```python
from build123d import *

# Parameters (mm, degrees)
SKETCH2_R           = 2.1
BOSS_EXTRUDE1_DEPTH = 746


with BuildPart() as part:
    # Sketch2 → Boss-Extrude1 (new body)
    with BuildSketch(Plane.XY):
        with BuildLine():
            Line((-0.1, 3.9), (0, 3.8))
            Line((0, 3.8), (0.1, 3.9))
            Line((0.1, 3.9), (2.840365134, 3.9))
            Line((2.840365134, 3.9), (5.5, 6.558825842))
            Line((5.5, 6.558825842), (5.5, 8.197505675))
            Line((5.5, 8.197505675), (2.89, 8.197505675))
            Line((2.89, 8.197505675), (2.89, 8.307505675))
            Line((2.89, 8.307505675), (4.348614357, 9.766120032))
            ThreePointArc((4.348614357, 9.766120032), (4.604908803, 9.937370505), (4.907228714, 9.997505675))
            Line((4.907228714, 9.997505675), (8.5, 9.997505675))
            ThreePointArc((8.5, 9.997505675), (9.560660172, 9.558165846), (10, 8.497505675))
            Line((10, 8.497505675), (10, 4.904734389))
            ThreePointArc((10, 4.904734389), (9.939864831, 4.602414477), (9.768614357, 4.346120032))
            Line((9.768614357, 4.346120032), (8.31, 2.887505675))
            Line((8.31, 2.887505675), (8.2, 2.887505675))
            Line((8.2, 2.887505675), (8.2, 5.497505675))
            Line((8.2, 5.497505675), (6.56, 5.497505675))
            Line((6.56, 5.497505675), (3.9, 2.83831481))
            Line((3.9, 2.83831481), (3.9, 0.1))
            Line((3.9, 0.1), (3.8, 0))
            Line((3.8, 0), (3.9, -0.1))
            Line((3.9, -0.1), (3.9, -2.84))
            Line((3.9, -2.84), (6.56, -5.5))
            Line((6.56, -5.5), (8.2, -5.5))
            Line((8.2, -5.5), (8.2, -2.89))
            Line((8.2, -2.89), (8.31, -2.89))
            Line((8.31, -2.89), (9.765685425, -4.345685425))
            ThreePointArc((9.765685425, -4.345685425), (9.939103626, -4.605224104), (10, -4.91137085))
            Line((10, -4.91137085), (10, -15.08862915))
            ThreePointArc((10, -15.08862915), (9.939103626, -15.394775896), (9.765685425, -15.654314575))
            Line((9.765685425, -15.654314575), (8.31, -17.11))
            Line((8.31, -17.11), (8.2, -17.11))
            Line((8.2, -17.11), (8.2, -14.5))
            Line((8.2, -14.5), (6.56, -14.5))
            Line((6.56, -14.5), (3.9, -17.16))
            Line((3.9, -17.16), (3.9, -19.9))
            Line((3.9, -19.9), (3.8, -20))
            Line((3.8, -20), (3.9, -20.1))
            Line((3.9, -20.1), (3.9, -22.83831481))
            Line((3.9, -22.83831481), (6.56, -25.497505675))
            Line((6.56, -25.497505675), (8.2, -25.497505675))
            Line((8.2, -25.497505675), (8.2, -22.887505675))
            Line((8.2, -22.887505675), (8.31, -22.887505675))
            Line((8.31, -22.887505675), (9.768614357, -24.346120032))
            ThreePointArc((9.768614357, -24.346120032), (9.939864831, -24.602414477), (10, -24.904734389))
            Line((10, -24.904734389), (10, -28.497505675))
            ThreePointArc((10, -28.497505675), (9.560660172, -29.558165846), (8.5, -29.997505675))
            Line((8.5, -29.997505675), (4.907228714, -29.997505675))
            ThreePointArc((4.907228714, -29.997505675), (4.604908803, -29.937370505), (4.348614357, -29.766120032))
            Line((4.348614357, -29.766120032), (2.89, -28.307505675))
            Line((2.89, -28.307505675), (2.89, -28.197505675))
            Line((2.89, -28.197505675), (5.5, -28.197505675))
            Line((5.5, -28.197505675), (5.5, -26.558825842))
            Line((5.5, -26.558825842), (2.840365134, -23.9))
            Line((2.840365134, -23.9), (0.1, -23.9))
            Line((0.1, -23.9), (0, -23.8))
            Line((0, -23.8), (-0.1, -23.9))
            Line((-0.1, -23.9), (-2.840365134, -23.9))
            Line((-2.840365134, -23.9), (-5.5, -26.558825842))
            Line((-5.5, -26.558825842), (-5.5, -28.197505675))
            Line((-5.5, -28.197505675), (-2.89, -28.197505675))
            Line((-2.89, -28.197505675), (-2.89, -28.307505675))
            Line((-2.89, -28.307505675), (-4.348614357, -29.766120032))
            ThreePointArc((-4.348614357, -29.766120032), (-4.604908803, -29.937370505), (-4.907228714, -29.997505675))
            Line((-4.907228714, -29.997505675), (-8.5, -29.997505675))
            ThreePointArc((-8.5, -29.997505675), (-9.560660172, -29.558165846), (-10, -28.497505675))
            Line((-10, -28.497505675), (-10, -24.904734389))
            ThreePointArc((-10, -24.904734389), (-9.939864831, -24.602414477), (-9.768614357, -24.346120032))
            Line((-9.768614357, -24.346120032), (-8.31, -22.887505675))
            Line((-8.31, -22.887505675), (-8.2, -22.887505675))
            Line((-8.2, -22.887505675), (-8.2, -25.497505675))
            Line((-8.2, -25.497505675), (-6.56, -25.497505675))
            Line((-6.56, -25.497505675), (-3.9, -22.83831481))
            Line((-3.9, -22.83831481), (-3.9, -20.1))
            Line((-3.9, -20.1), (-3.8, -20))
            Line((-3.8, -20), (-3.9, -19.9))
            Line((-3.9, -19.9), (-3.9, -17.16))
            Line((-3.9, -17.16), (-6.56, -14.5))
            Line((-6.56, -14.5), (-8.2, -14.5))
            Line((-8.2, -14.5), (-8.2, -17.11))
            Line((-8.2, -17.11), (-8.31, -17.11))
            Line((-8.31, -17.11), (-9.765685425, -15.654314575))
            ThreePointArc((-9.765685425, -15.654314575), (-9.939103626, -15.394775896), (-10, -15.08862915))
            Line((-10, -15.08862915), (-10, -4.91137085))
            ThreePointArc((-10, -4.91137085), (-9.939103626, -4.605224104), (-9.765685425, -4.345685425))
            Line((-9.765685425, -4.345685425), (-8.31, -2.89))
            Line((-8.31, -2.89), (-8.2, -2.89))
            Line((-8.2, -2.89), (-8.2, -5.5))
            Line((-8.2, -5.5), (-6.56, -5.5))
            Line((-6.56, -5.5), (-3.9, -2.84))
            Line((-3.9, -2.84), (-3.9, -0.1))
            Line((-3.9, -0.1), (-3.8, 0))
            Line((-3.8, 0), (-3.9, 0.1))
            Line((-3.9, 0.1), (-3.9, 2.83831481))
            Line((-3.9, 2.83831481), (-6.56, 5.497505675))
            Line((-6.56, 5.497505675), (-8.2, 5.497505675))
            Line((-8.2, 5.497505675), (-8.2, 2.887505675))
            Line((-8.2, 2.887505675), (-8.31, 2.887505675))
            Line((-8.31, 2.887505675), (-9.768614357, 4.346120032))
            ThreePointArc((-9.768614357, 4.346120032), (-9.939864831, 4.602414477), (-10, 4.904734389))
            Line((-10, 4.904734389), (-10, 8.497505675))
            ThreePointArc((-10, 8.497505675), (-9.560660172, 9.558165846), (-8.5, 9.997505675))
            Line((-8.5, 9.997505675), (-4.907228714, 9.997505675))
            ThreePointArc((-4.907228714, 9.997505675), (-4.604908803, 9.937370505), (-4.348614357, 9.766120032))
            Line((-4.348614357, 9.766120032), (-2.89, 8.307505675))
            Line((-2.89, 8.307505675), (-2.89, 8.197505675))
            Line((-2.89, 8.197505675), (-5.5, 8.197505675))
            Line((-5.5, 8.197505675), (-5.5, 6.558825842))
            Line((-5.5, 6.558825842), (-2.840365134, 3.9))
            Line((-2.840365134, 3.9), (-0.1, 3.9))
        make_face()
        Circle(SKETCH2_R, mode=Mode.SUBTRACT)
        with Locations(Location((0, -20, 0), (0, 0, 180))):
            Circle(SKETCH2_R, mode=Mode.SUBTRACT)
        Polygon((-7.66, 6.567505675), (-6.57, 7.657505675), (-6.57, 8.197505675), (-8.2, 8.197505675), (-8.2, 6.567505675), align=None, mode=Mode.SUBTRACT)
        Polygon((-0.1, -3.9), (0, -3.8), (0.1, -3.9), (2.840365134, -3.9), (6.24, -7.299634866), (8.2, -7.299634866), (8.2, -12.700365134), (6.24, -12.700365134), (2.840365134, -16.1), (0.1, -16.1), (0, -16.2), (-0.1, -16.1), (-2.840365134, -16.1), (-6.24, -12.700365134), (-8.2, -12.700365134), (-8.2, -7.299634866), (-6.24, -7.299634866), (-2.840365134, -3.9), align=None, mode=Mode.SUBTRACT)
        Polygon((8.2, 6.567505675), (7.66, 6.567505675), (6.57, 7.657505675), (6.57, 8.197505675), (8.2, 8.197505675), align=None, mode=Mode.SUBTRACT)
        Polygon((7.66, -26.567505675), (6.57, -27.657505675), (6.57, -28.197505675), (8.2, -28.197505675), (8.2, -26.567505675), align=None, mode=Mode.SUBTRACT)
        Polygon((-8.2, -26.567505675), (-7.66, -26.567505675), (-6.57, -27.657505675), (-6.57, -28.197505675), (-8.2, -28.197505675), align=None, mode=Mode.SUBTRACT)
    extrude(amount=-BOSS_EXTRUDE1_DEPTH)


solid = part.part
```
Geometry: final body of the model. Coordinates: model frame, mm. Coordinates: 2 decimals unless noted, no trailing zeros. Use a Markdown table: item, result. Add a question column.
(1) Section query A-A, the plane z = -240. State how many separate pieces and enclosed holes the cut face has, plus the area to 3 significant figures.
(2) Line query: line 1 along Y through (x, z) = (0, -558); line 2 along X through (y, z) = (8, -442.5); line 3 along X through (y, z) = (-11.5, -411.5). Output: solid intervals per line, ascending.
(3) Pin query (flat end, axial travel): pin 1 Ø3 at (y, z) = (-21.5, -325.5) entering from -X; pin 2 Ø2 at (x, z) = (-1, -528.5) entering from +Y; pin 3 Ø1 at (x, z) = (-3.5, -314) entering from -Y. Return the tip coordinate at first contact, or that it passes through.
Answer:
| question | item | result |
|---|---|---|
| 1 | separate pieces | 1 |
| 1 | enclosed holes | 7 |
| 1 | area | 291 mm^2 |
| 2 | line 1 | y = -23.8 to -22.1, -17.9 to -16.2, -3.8 to -2.1, 2.1 to 3.8 |
| 2 | line 2 | x = -10 to -8.2, -6.57 to -5.5, 5.5 to 6.57, 8.2 to 10 |
| 2 | line 3 | x = -10 to -8.2, 8.2 to 10 |
| 3 | pin 1 | stops at x = -8.42 |
| 3 | pin 2 | stops at y = 3.9 |
| 3 | pin 3 | stops at y = -29.42 |
